from build123d import *

# Parameters (mm, degrees)
SALIENTE_EXTRUIR1_DEPTH      = 50
SALIENTE_EXTRUIR3_DEPTH      = 1
SALIENTE_EXTRUIR3_DEPTH_BACK = 11
CROQUIS8_R                   = 5.1
CORTAR_EXTRUIR1_DEPTH        = 20


with BuildPart() as part:
    # Croquis1 → Saliente-Extruir1 (new body)
    with BuildSketch(Plane.XY):
        with BuildLine():
            Line((-84.492533904, -6.921751872), (-44.492533904, -6.921751872))
            Line((-44.492533904, -6.921751872), (-44.492533904, -5.660932217))
            ThreePointArc((-44.492533904, -5.660932217), (-44.785427123, -4.953825435), (-45.492533904, -4.660932217))
            Line((-45.492533904, -4.660932217), (-59.602097354, -4.660932217))
            Line((-59.602097354, -4.660932217), (-59.602097354, 10.986403293))
            Line((-59.602097354, 10.986403293), (-55.79772825, 21.438821499))
            ThreePointArc((-55.79772825, 21.438821499), (-55.831113084, 22.203459904), (-56.395400728, 22.720534263))
            Line((-56.395400728, 22.720534263), (-58.274785969, 23.40457455))
            ThreePointArc((-58.274785969, 23.40457455), (-59.039424374, 23.371189716), (-59.556498733, 22.806902073))
            Line((-59.556498733, 22.806902073), (-69.073702494, -3.341400356))
            ThreePointArc((-69.073702494, -3.341400356), (-69.439818678, -3.818532257), (-70.013395115, -3.999380213))
            Line((-70.013395115, -3.999380213), (-79.590995067, -3.999380213))
            ThreePointArc((-79.590995067, -3.999380213), (-80.410147111, -3.572956649), (-80.530687688, -2.657360069))
            Line((-80.530687688, -2.657360069), (-77.297371662, 6.226102703))
            ThreePointArc((-77.297371662, 6.226102703), (-77.330756495, 6.990741108), (-77.895044139, 7.507815467))
            Line((-77.895044139, 7.507815467), (-78.855503706, 7.857394161))
            ThreePointArc((-78.855503706, 7.857394161), (-79.609989894, 7.828674516), (-80.129339821, 7.280632657))
            Line((-80.129339821, 7.280632657), (-84.424349875, -3.746691195))
            ThreePointArc((-84.424349875, -3.746691195), (-84.475340083, -3.924982082), (-84.492533904, -4.109622312))
            Line((-84.492533904, -4.109622312), (-84.492533904, -6.921751872))
        make_face()
    extrude(amount=SALIENTE_EXTRUIR1_DEPTH)

    # Croquis5 → Saliente-Extruir3 (add, two sides)
    with BuildSketch(Plane(origin=(-12.054515952, -30.949648451, 0), x_dir=(0, 0, 1), z_dir=(-0.362931117, -0.931815971, 0))) as saliente_extruir3_sk:
        Polygon((17.5, 77.308166751), (30.522755533, 88.235556115), (45.522755533, 88.235556115), (32.5, 77.308166751), align=None)
    extrude(amount=SALIENTE_EXTRUIR3_DEPTH)
    extrude(saliente_extruir3_sk.sketch, amount=-SALIENTE_EXTRUIR3_DEPTH_BACK)

    # Croquis8 → Cortar-Extruir1 (cut)
    with BuildSketch(Plane(origin=(-54.858231018, 21.366621399, 70.161379414), x_dir=(0.800779124, 0.174492436, 0.572979218), z_dir=(-0.598959761, 0.233287625, 0.766044443))):
        with Locations((-51.412419204, -5.511649837)):
            Circle(CROQUIS8_R)
    extrude(amount=-CORTAR_EXTRUIR1_DEPTH, mode=Mode.SUBTRACT)


solid = part.part
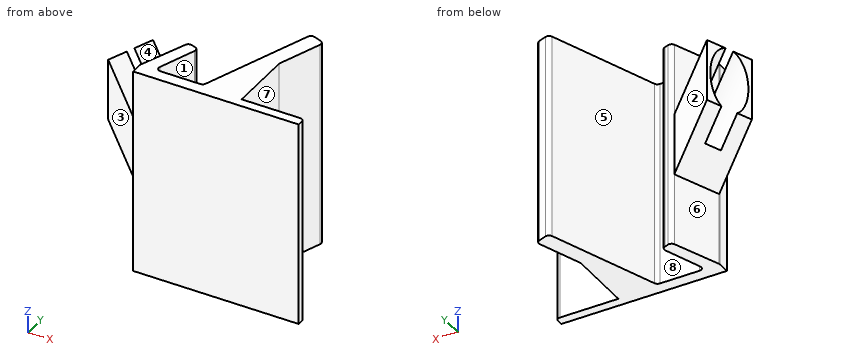
CAD build for the part. Positions are in the model's coordinates, mm. Face numbers are marked on the shaded views. A direction names the side the tool comes from. Give positions to 0.01 mm unless a question says otherwise; leave off trailing zeros. Loops run counter-clockwise (first coordinate to the right, second up) from the corner with the lowest first, then second, coordinate; pieces in that order, holes last. Notation, with made-up numbers: M 8,-4.5 L 27,-4.5 A19 cw 27,22.5 Z; hole C -7,-8 d8. An arc over 180 degrees is marked long. One line per question, with ' | ' between items. Start each with the question number.
1. Probe L1, parallel to Y at x = -77, z = 29; L2, parallel to Z at x = -91, y = 1.5; L3, parallel to Y at x = -50.5, z = 40.5. List the from-to ranges inside material, lowest first. Write a range as from..to.
2. 3-axis set-ups, long thin cutter, end or side, ignore diameter. For the marked faces 5, 6, 7 and 8: which of +Z, -Z, +X, -X, +Y, -Y reach the whole face in a straight line?
3. Saw through at C-C on y = 16. Give the cut face in (x, z), plus the area to 3 significant figures.
4. Two-plate mould, pull along Y, no slides. Class the marked faces 1, 2, 3 and 4: pulls with the +Y half, pulls with the -Y half, needs draft (parallel to the pull), parting line crosses it, or undercut.
5. Saw through at A-A on x = -74. Give the cut face in (y, z).
6. Flat gauge pins, fed straight in: pin 1 (10 mm diameter, centred on y = -2.5, z = 25.5, fed in from -X); pin 2 (6 mm diameter, centred on y = 1.5, z = 29.5, fed in from +X); pin 3 (5 mm diameter, centred on x = -77, z = 20, fed in from +Y); pin 4 (12 mm diameter, centred on x = -65, y = 18, fed in from -Z). Where does each tip first touch, or does it go through?
7. Saw through at D-D on z = 23. Give the cut face in (x, y), plus the area to 3 significant figures.
8. Saw through at B-B on z = 40.5. State how many separate pieces and enclosed holes the cut face has, plus the area to 3 significant figures.
Result sheet:
1) L1: y = -6.92..-4 | L2: z = 27.07..28.4, 40.19..42.07 | L3: y = -6.92..-4.66
2) face 5: +Z, -Z, +Y | face 6: -Z, -X, +Y | face 7: +Z, -Z, +X | face 8: +Z, -Z
3) outline: M -62.03,0 L -57.78,0 L -57.78,50 L -62.03,50 Z | area: 213 mm^2
4) face 1: undercut | face 2: pulls with the +Y half | face 3: pulls with the -Y half | face 4: undercut
5) outline: M -6.92,0 L -4,0 L -4,50 L -6.92,50 Z
6) pin 1: stops at x = -94.12 | pin 2: stops at x = -59.6 | pin 3: stops at y = 7.92 | pin 4: stops at z = 0
7) outline: M -88.75,-2.15 L -84.45,-3.82 L -84.42,-3.75 A1 ccw -84.49,-4.11 L -84.49,-6.92 L -44.49,-6.92 L -44.49,-5.66 A1 ccw -45.49,-4.66 L -59.6,-4.66 L -59.6,10.99 L -55.8,21.44 A1 ccw -56.4,22.72 L -58.27,23.4 A1 ccw -59.56,22.81 L -69.07,-3.34 A1 cw -70.01,-4 L -79.59,-4 A1 cw -80.53,-2.66 L -77.3,6.23 A1 ccw -77.9,7.51 L -78.86,7.86 A1 ccw -80.13,7.28 L -80.1,7.36 L -84.4,9.03 Z | area: 357 mm^2
8) separate pieces: 3 | enclosed holes: 0 | area: 322 mm^2
